from build123d import *

# Parameters (mm, degrees)
UPPER_START = 67
UPPER_DEPTH = 6.2
NECK_START  = 65.5
NECK_DEPTH  = 1.7
BODY_START  = 59
BODY_DEPTH  = 6.5
STEM_START  = 73.2
STEM_DEPTH  = 3.6


with BuildPart() as part:
    # Sketch1 → Upper (new body)
    with BuildSketch(Plane(origin=(0, 0, 0), x_dir=(1, 0, 0), z_dir=(0, 1, 0)).offset(UPPER_START)):
        with BuildLine():
            Line((-7.2, 89.3), (7.2, 89.3))
            ThreePointArc((7.2, 89.3), (7.624264069, 89.124264069), (7.8, 88.7))
            Line((7.8, 88.7), (7.8, 74.3))
            ThreePointArc((7.8, 74.3), (7.624264069, 73.875735931), (7.2, 73.7))
            Line((7.2, 73.7), (-7.2, 73.7))
            ThreePointArc((-7.2, 73.7), (-7.624264069, 73.875735931), (-7.8, 74.3))
            Line((-7.8, 74.3), (-7.8, 88.7))
            ThreePointArc((-7.8, 88.7), (-7.624264069, 89.124264069), (-7.2, 89.3))
        make_face()
    extrude(amount=UPPER_DEPTH)

    # Sketch2 → Neck (add)
    with BuildSketch(Plane(origin=(0, 0, 0), x_dir=(1, 0, 0), z_dir=(0, 1, 0)).offset(NECK_START)):
        with BuildLine():
            Line((-6.55, 88.45), (6.55, 88.45))
            ThreePointArc((6.55, 88.45), (6.832842712, 88.332842712), (6.95, 88.05))
            Line((6.95, 88.05), (6.95, 74.95))
            ThreePointArc((6.95, 74.95), (6.832842712, 74.667157288), (6.55, 74.55))
            Line((6.55, 74.55), (-6.55, 74.55))
            ThreePointArc((-6.55, 74.55), (-6.832842712, 74.667157288), (-6.95, 74.95))
            Line((-6.95, 74.95), (-6.95, 88.05))
            ThreePointArc((-6.95, 88.05), (-6.832842712, 88.332842712), (-6.55, 88.45))
        make_face()
    extrude(amount=NECK_DEPTH)

    # Sketch3 → Body (add)
    with BuildSketch(Plane(origin=(0, 0, 0), x_dir=(1, 0, 0), z_dir=(0, 1, 0)).offset(BODY_START)):
        with BuildLine():
            Line((-6.9, 89), (6.9, 89))
            ThreePointArc((6.9, 89), (7.324264069, 88.824264069), (7.5, 88.4))
            Line((7.5, 88.4), (7.5, 74.6))
            ThreePointArc((7.5, 74.6), (7.324264069, 74.175735931), (6.9, 74))
            Line((6.9, 74), (-6.9, 74))
            ThreePointArc((-6.9, 74), (-7.324264069, 74.175735931), (-7.5, 74.6))
            Line((-7.5, 74.6), (-7.5, 88.4))
            ThreePointArc((-7.5, 88.4), (-7.324264069, 88.824264069), (-6.9, 89))
        make_face()
    extrude(amount=BODY_DEPTH)

    # Sketch4 → Stem (add)
    with BuildSketch(Plane(origin=(0, 0, 0), x_dir=(1, 0, 0), z_dir=(0, 1, 0)).offset(STEM_START)):
        with BuildLine():
            Line((-3.2, 85.1), (3.2, 85.1))
            ThreePointArc((3.2, 85.1), (3.482842712, 84.982842712), (3.6, 84.7))
            Line((3.6, 84.7), (3.6, 78.3))
            ThreePointArc((3.6, 78.3), (3.482842712, 78.017157288), (3.2, 77.9))
            Line((3.2, 77.9), (-3.2, 77.9))
            ThreePointArc((-3.2, 77.9), (-3.482842712, 78.017157288), (-3.6, 78.3))
            Line((-3.6, 78.3), (-3.6, 84.7))
            ThreePointArc((-3.6, 84.7), (-3.482842712, 84.982842712), (-3.2, 85.1))
        make_face()
    extrude(amount=STEM_DEPTH)


solid = part.part
Input: part model. Units: mm. Frame: model coordinates. A direction names the side the tool comes from. Round coordinates to 2 decimals unless told otherwise and drop trailing zeros. Loops run counter-clockwise (first coordinate to the right, second up) from the corner with the lowest first, then second, coordinate; pieces in that order, holes last. Notation, with made-up numbers: (11, -11.75) -> (39, -11.75) arc R32 cw to (39, 16.25) -> close; hole circle Ø6 at (13.25, 55.25). An arc over 180 degrees is marked (long way). Answer as a JSON object with one key per item and string values. Group by question number.
1) Ray query, L1, parallel to Y at x = -4.5, z = -88.5; L2, parallel to Y at x = -4.5, z = -82; L3, parallel to Z at x = -6, y = 61.75. Return the intervals inside material, ascending.
2) Reachability of faces 1 (the flat face through (-6.95, 66, -81)), 2 (the flat face through (0, 66, -74.55)), 3 (the flat face through (0, 75, -77.9)) from +Z, -Z, +X, -X, +Y, -Y: full face, straight path, thin tool, end or side. Return the list, or none.
3) Section query B-B on y = 73.5. Output: boundary loops of the cut face in (x, z).
4) Section query D-D on z = -87.25. Output: boundary loops of the cut face in (x, y).
5) Draft query along Y for faces 4 (the flat face through (4, 73.2, -85)), 5 (the flat face through (6.95, 66, -82)), 6 (the flat face through (7.8, 70, -82)). Return one class per face: +Y half, -Y half, draft (parallel to the pull), parting line (faces both ways), or undercut.
6) Pin query (flat end, axial travel): pin 1 (1.1 mm diameter, centred on y = 75.5, z = -81, fed in from +X); pin 2 (7 mm diameter, centred on y = 63, z = -81, fed in from -X); pin 3 (1.2 mm diameter, centred on x = -1.5, y = 66, fed in from -Z). Return the tip coordinate at first contact, or that it passes through.
7) Section query A-A on z = -78.75. Output: boundary loops of the cut face in (x, y), plus the area to 3 significant figures.
8) Section query C-C on x = 4.5. Output: boundary loops of the cut face in (y, z).
Reply:
{
 "1": {"L1": "y = 59 to 65.5, 67 to 73.2", "L2": "y = 59 to 73.2", "L3": "z = -89 to -74"},
 "2": {"face 1": "+Z, -Z, -X", "face 2": "+Z, +X, -X", "face 3": "+Z, +X, -X, +Y"},
 "3": {"outline": "(-3.6, -84.7) arc R0.4 ccw to (-3.2, -85.1) -> (3.2, -85.1) arc R0.4 ccw to (3.6, -84.7) -> (3.6, -78.3) arc R0.4 ccw to (3.2, -77.9) -> (-3.2, -77.9) arc R0.4 ccw to (-3.6, -78.3) -> close"},
 "4": {"outline": "(-7.8, 67) -> (-6.95, 67) -> (-6.95, 65.5) -> (-7.5, 65.5) -> (-7.5, 59) -> (7.5, 59) -> (7.5, 65.5) -> (6.95, 65.5) -> (6.95, 67) -> (7.8, 67) -> (7.8, 73.2) -> (-7.8, 73.2) -> close"},
 "5": {"face 4": "+Y half", "face 5": "undercut", "face 6": "draft"},
 "6": {"pin 1": "stops at x = 3.6", "pin 2": "stops at x = -7.5", "pin 3": "stops at z = -89"},
 "7": {"outline": "(-7.8, 67) -> (-6.95, 67) -> (-6.95, 65.5) -> (-7.5, 65.5) -> (-7.5, 59) -> (7.5, 59) -> (7.5, 65.5) -> (6.95, 65.5) -> (6.95, 67) -> (7.8, 67) -> (7.8, 73.2) -> (3.6, 73.2) -> (3.6, 76.8) -> (-3.6, 76.8) -> (-3.6, 73.2) -> (-7.8, 73.2) -> close", "area": "241 mm2"},
 "8": {"outline": "(59, -89) -> (65.5, -89) -> (65.5, -88.45) -> (67, -88.45) -> (67, -89.3) -> (73.2, -89.3) -> (73.2, -73.7) -> (67, -73.7) -> (67, -74.55) -> (65.5, -74.55) -> (65.5, -74) -> (59, -74) -> close"}
}
